Check sheet for the modelled part. Datum: model origin and axes. Units: mm. Face numbers are marked on the shaded views. A direction names the side the tool comes from. Give positions to 0.01 mm unless a question says otherwise; leave off trailing zeros. Order: outer loops, then holes, each group sorted by start corner. A loop starts at its lowest first (then second) coordinate and runs counter-clockwise, first axis right, second up.
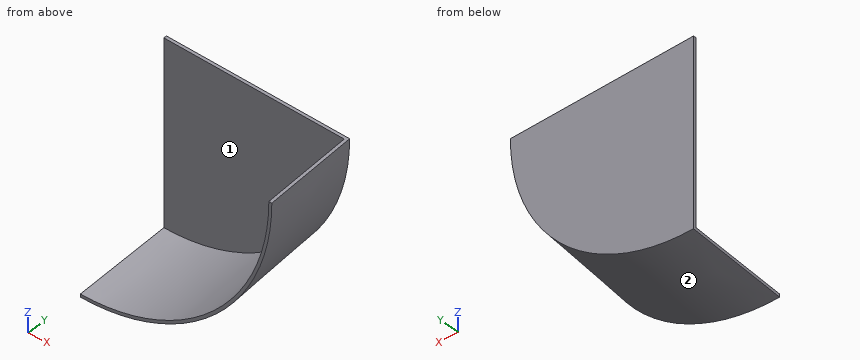
Autodesk Inventor part; units mm, degrees
ref_plane "YZ Plane" through (0, 0, 0) normal (1, 0, 0) x (0, 1, 0)
ref_plane "XZ Plane" through (0, 0, 0) normal (0, 1, 0) x (-1, 0, 0)
ref_plane "XY Plane" through (0, 0, 0) normal (0, 0, 1) x (1, 0, 0)
sketch "Sketch1" plane through (0, 0, 0) normal (1, 0, 0) x (0, 1, 0)
  line L0 (52.2781, 123.0082) -> (49.1031, 123.0082)
  line L1 (-49.3219, -80.1918) -> (-49.3219, -77.0168)
  line L2 (-49.3219, -77.0168) -> (49.1031, -68.4058)
  line L3 (52.2781, -68.128) -> (52.2781, -71.303)
  line L4 (-49.3219, -80.1918) -> (52.2781, -71.303)
  line L5 (52.2781, -68.128) -> (52.2781, 123.0082)
  line L6 (49.1031, 123.0082) -> (49.1031, -68.4058)
  point P0 (0, 0)
  dimension "d0" = 203.2
  dimension "d1" = 3.175
  dimension "d2" = 95
  dimension "d3" = 101.6
  dimension "d4" = 180
  dimension "d5" = 3.175
revolve "Revolution1" add sketch "Sketch1" angle 90 about axis through (0, 52.2781, 123.0082) along (0, -1, 0)
properties part number "QuarterTop"
(1) Cross-section at A-A on y = -4. Enter the section's corners in (x, z).
Response values:
outline: (0, -76.23) arc R199.23 ccw to (199.23, 123.01) - (196.06, 123.01) arc R196.06 cw to (0, -73.05) - close
(2) Set-up check for the marked faces 1 and 2: record each of +Z, -Z, +X, -X, +Y, -Y from which the full face is reachable in a straight line by a thin tool's end or side.
Response values:
face 1: +Z, -X, -Y
face 2: -Z, +X, +Y
(3) Cross-section at B-B on y = -31.5. Enter the section's corners in (x, z).
Response values:
outline: (0, -78.63) arc R201.64 ccw to (201.64, 123.01) - (198.47, 123.01) arc R198.47 cw to (0, -75.46) - close
(4) Gauge pin test, flat ends, axial feed: pin 1 Ø10 at (x, y) = (105.5, -2) entering from -Z; pin 2 Ø1 at (y, z) = (-2.5, -18) entering from +X; pin 3 Ø1.5 at (y, z) = (23.5, 57) entering from +X (3 decimals). Record the tip position at first contact, or that the pin passes through.
Response values:
pin 1: stops at z = -48.86
pin 2: stops at x = 141.07
pin 3: stops at x = 185.705
(5) Material ranges on L1, parallel to Y at x = 97, z = 19; L2, parallel to Z at x = 34, y = 6.5; L3, parallel to Z at x = 72, y = 45, recorded low to high.
Response values:
L1: y = 49.1 to 52.28
L2: z = -72.37 to -69.15
L3: z = -58.16 to -54.74
